Part model, mm, in its own coordinate system. Face numbers are marked on the shaded views. Round coordinates to 2 decimals unless told otherwise and drop trailing zeros. Order: outer loops, then holes, each group sorted by start corner. A loop starts at its lowest first (then second) coordinate and runs counter-clockwise, first axis right, second up. Notation, with made-up numbers: M 14.25,54 L 41.25,54 A29 ccw 41.25,93 Z; hole C 70.5,46 d3. An arc over 180 degrees is marked long. One line per question, with ' | ' between items.
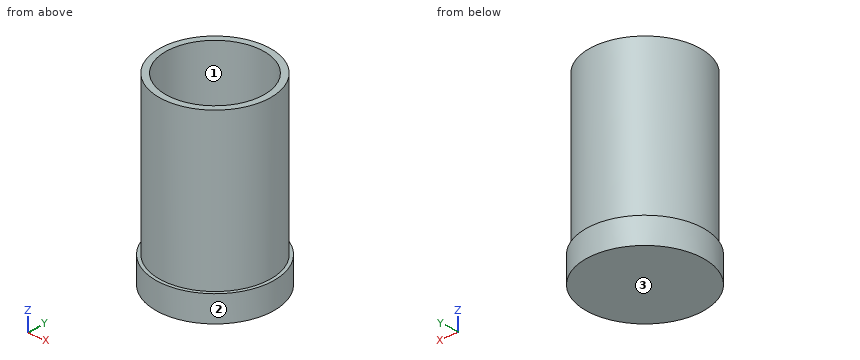
from build123d import *

# Parameters (mm, degrees)
F0_W = 3.175
F0_H = 19.05


with BuildPart() as f1:
    # F0 (on Front) → F1 (revolve)
    with BuildSketch(Plane.XZ):
        Polygon((-57.15, 0), (0, 0), (0, 6.35), (-47.625, 6.35), (-53.975, 6.35), (-57.15, 6.35), align=None)
        with Locations((-55.5625, 15.875)):
            Rectangle(F0_W, F0_H)
        Polygon((-53.975, 6.35), (-47.625, 6.35), (-47.625, 177.8), (-53.975, 177.8), (-53.975, 25.4), align=None)
    revolve(axis=Axis((0, 0, 3.175), (0, 0, 1)))


solid = f1.part
1) Drop flat-ended pins along their axis: pin 1 (4 mm diameter, centred on x = 28.5, z = 34, fed in from -Y); pin 2 (1 mm diameter, centred on y = 7.5, z = 88, fed in from +X); pin 3 (10 mm diameter, centred on y = -4.5, z = 83.5, fed in from -X) (3 decimals); pin 4 (1 mm diameter, centred on x = -19.5, y = -31.5, fed in from -Z). Give the stop position or say it passes through.
The answers:
pin 1: stops at y = -47.02 | pin 2: stops at x = 53.52 | pin 3: stops at x = -53.975 | pin 4: stops at z = 0
2) Two-plate mould, pull along Y, no slides. Class the marked faces 1, 2 and 3: released by +Y, released by -Y, zero draft, split by the parting line, or undercut.
The answers:
face 1: undercut | face 2: split by the parting line | face 3: zero draft
3) Saw through at A-A (x = 0). List the corners of the cut face in (y, z) (3 decimals).
The answers:
outline: M -57.15,0 L 57.15,0 L 57.15,25.4 L 53.975,25.4 L 53.975,177.8 L 47.625,177.8 L 47.625,6.35 L -47.625,6.35 L -47.625,177.8 L -53.975,177.8 L -53.975,25.4 L -57.15,25.4 Z
4) Saw through at C-C (z = 148). List the corners of the cut face in (x, y) (3 decimals), plus the area to 3 significant figures.
The answers:
outline: C 0,0 d107.95; hole C 0,0 d95.25 | area: 2,030 mm²
5) Probe line 1 (X direction, y = 0, z = 86) (3 decimals); line 2 (Z direction, x = -17, y = -10). List the from-to ranges inside material, lowest first. Write a range as [from, to].
The answers:
line 1: x = [-53.975, -47.625], [47.625, 53.975] | line 2: z = [0, 6.35]
